from build123d import *

# Parameters (mm, degrees)
SKETCH1_W           = 40
SKETCH1_H           = 12
SKETCH1_W_2         = 50
SKETCH1_H_2         = 20
SKETCH1_W_3         = 20
SKETCH1_H_3         = 4.5
BOSS_EXTRUDE1_DEPTH = 4.5
FILLET1_R           = 4


with BuildPart() as part:
    # Sketch1 → Boss-Extrude1 (new body)
    with BuildSketch(Plane(origin=(0, 0, 0), x_dir=(0, 0, -1), z_dir=(1, 0, 0))):
        Polygon((0, 0), (0, 5), (0, 45), (0, 50), (0, 90), (0, 95), (0, 115), (90, 115), (90, 45), (90, 5), (90, 0), align=None)
        with Locations((45, 105)):
            Rectangle(SKETCH1_W, SKETCH1_H, mode=Mode.SUBTRACT)
        with Locations((45, 70)):
            Rectangle(SKETCH1_W, SKETCH1_H, mode=Mode.SUBTRACT)
        with Locations((45, 25)):
            Rectangle(SKETCH1_W_2, SKETCH1_H_2, mode=Mode.SUBTRACT)
        with Locations((65, 92.25)):
            Rectangle(SKETCH1_W_3, SKETCH1_H_3, mode=Mode.SUBTRACT)
        with Locations((25, 92.25)):
            Rectangle(SKETCH1_W_3, SKETCH1_H_3, mode=Mode.SUBTRACT)
        with Locations((65, 47.5)):
            Rectangle(SKETCH1_W_3, SKETCH1_H_3, mode=Mode.SUBTRACT)
        with Locations((25, 47.5)):
            Rectangle(SKETCH1_W_3, SKETCH1_H_3, mode=Mode.SUBTRACT)
        with Locations((65, 8)):
            Rectangle(SKETCH1_W_3, SKETCH1_H_3, mode=Mode.SUBTRACT)
        with Locations((25, 8)):
            Rectangle(SKETCH1_W_3, SKETCH1_H_3, mode=Mode.SUBTRACT)
    extrude(amount=BOSS_EXTRUDE1_DEPTH)

    # Fillet1
    fillet1_edges = [part.edges().sort_by_distance(p)[0] for p in [
        (2.25, 76, -65),
        (2.25, 76, -25),
        (2.25, 35, -70),
        (2.25, 35, -20),
        (2.25, 111, -65),
        (2.25, 111, -25),
    ]]
    fillet(fillet1_edges, radius=FILLET1_R)


solid = part.part
Geometry check sheet. Reference: the model listing, model coordinates, mm. A direction names the side the tool comes from. Round coordinates to 2 decimals unless told otherwise and drop trailing zeros. Write each loop counter-clockwise with the first axis right and the second up, starting at its lowest first coordinate (ties: lowest second). Pieces come first, ordered by that corner, then holes.
Item 1: Access from +Z, -Z, +X, -X, +Y, -Y to the whole of each face (thin tool, end or side, straight path). Record for faces 4 (the face through (0, 58, -46)), 5 (the face through (2, 8, -35)).
Determined:
face 4: +Z, -Z, -X, +Y, -Y
face 5: +X, -X
Item 2: Material ranges on line 1 along Z through (x, y) = (3.15, 8); line 2 along Y through (x, z) = (4.3, -51.5); line 3 along Y through (x, z) = (2.15, -18.5), recorded low to high.
Determined:
line 1: z = -90 to -75, -55 to -35, -15 to 0
line 2: y = 0 to 15, 35 to 64, 76 to 99, 111 to 115
line 3: y = 0 to 5.75, 10.25 to 45.25, 49.75 to 90, 94.5 to 115
Item 3: Section check C-C (z = -43). Record the boundary of the cut face in (x, y), plus the area to 4 significant figures.
Determined:
outline: (0, 0) - (4.5, 0) - (4.5, 15) - (0, 15) - close; (0, 35) - (4.5, 35) - (4.5, 64) - (0, 64) - close; (0, 76) - (4.5, 76) - (4.5, 99) - (0, 99) - close; (0, 111) - (4.5, 111) - (4.5, 115) - (0, 115) - close
area: 319.5 mm2
Item 4: Mould release check, pull along Z, two halves, no side actions. Record for faces 1 (the face through (2, 57, -90)), 2 (the face through (2, 15, -45)), 3 (the face through (2, 0, -46)): +Z half, -Z half, draft (parallel to the pull), parting line (faces both ways), or undercut.
Determined:
face 1: -Z half
face 2: undercut
face 3: draft
Item 5: Section check A-A (z = -73.5). Record the boundary of the cut face in (x, y), plus the area to 3 significant figures.
Determined:
outline: (0, 0) - (4.5, 0) - (4.5, 5.75) - (0, 5.75) - close; (0, 10.25) - (4.5, 10.25) - (4.5, 45.25) - (0, 45.25) - close; (0, 49.75) - (4.5, 49.75) - (4.5, 90) - (0, 90) - close; (0, 94.5) - (4.5, 94.5) - (4.5, 115) - (0, 115) - close
area: 457 mm2
Item 6: Section check B-B (x = 0.75). Give the number of separate pieces and of enclosed holes in the cut face, plus the area to 3 significant figures.
Determined:
separate pieces: 1
enclosed holes: 9
area: 7,870 mm2
